from build123d import *

# Parameters (mm, degrees)
SKETCH1_W                                        = 32
SKETCH1_H                                        = 60
BOSS_EXTRUDE1_DEPTH                              = 7
SKETCH2_W                                        = 51
SKETCH2_H                                        = 8.75
CUT_EXTRUDE1_DEPTH                               = 65.078077374
CUT_EXTRUDE2_DEPTH                               = 65.078077374
F_10_0_10_DIAMETER_HOLE1_D                       = 10
F_10_0_10_DIAMETER_HOLE1_DEPTH                   = 14
M4X0_7_TAPPED_HOLE1_D                            = 2.1
M4X0_7_TAPPED_HOLE1_DEPTH                        = 14
M4X0_7_TAPPED_HOLE1_CBORE_D                      = 4
M4X0_7_TAPPED_HOLE1_CBORE_DEPTH                  = 2
CBORE_FOR_M3_HEX_HEAD_MACHINE_SCREW1_D           = 3.2
CBORE_FOR_M3_HEX_HEAD_MACHINE_SCREW1_CBORE_D     = 10.2
CBORE_FOR_M3_HEX_HEAD_MACHINE_SCREW1_CBORE_DEPTH = 1
F_4_1_4_1_DIAMETER_HOLE1_D                       = 4.1
F_4_1_4_1_DIAMETER_HOLE1_DEPTH                   = 14
F_4_1_4_1_DIAMETER_HOLE2_D                       = 4.1
FILLET3_R                                        = 12
CUT_EXTRUDE3_DEPTH                               = 65.078077374
SKETCH24_W                                       = 59.877724024
SKETCH24_H                                       = 41.345566777
CUT_EXTRUDE4_DEPTH                               = 7


# Read off the part's stored shape, not the designer's step: Mirror1
with BuildPart() as part:
    # Sketch1 → Boss-Extrude1 (new body)
    with BuildSketch(Plane(origin=(-2, 0, 0), x_dir=(0, -1, 0), z_dir=(-1, 0, 0))):
        with Locations((-8, 29)):
            Rectangle(SKETCH1_W, SKETCH1_H)
    extrude(amount=-BOSS_EXTRUDE1_DEPTH)

    # Sketch2 → Cut-Extrude1 (cut, through all)
    with BuildSketch(Plane(origin=(5, 0, 0), x_dir=(0, 0, -1), z_dir=(1, 0, 0))):
        with Locations((-21.5, 19.625)):
            Rectangle(SKETCH2_W, SKETCH2_H)
    extrude(amount=-CUT_EXTRUDE1_DEPTH, mode=Mode.SUBTRACT)

    # Sketch3 → Cut-Extrude2 (cut, through all)
    with BuildSketch(Plane(origin=(5, 0, 0), x_dir=(0, 0, -1), z_dir=(1, 0, 0))):
        Polygon((4, 6.75), (-21, 6.75), (-23, 15.25), (4, 15.25), align=None)
    extrude(amount=-CUT_EXTRUDE2_DEPTH, mode=Mode.SUBTRACT)

    # Ø10.0 (10) Diameter Hole1
    with Locations(Plane.ZY.offset(2)):
        with Locations((28, 0)):
            Hole(F_10_0_10_DIAMETER_HOLE1_D / 2, depth=F_10_0_10_DIAMETER_HOLE1_DEPTH)

    # M4x0.7 Tapped Hole1
    with Locations(Plane.ZY.offset(2)):
        with Locations((38.968179165, 5), (51.718179165, -2.361215932), (51.718179165, 12.361215932)):
            CounterBoreHole(M4X0_7_TAPPED_HOLE1_D / 2, M4X0_7_TAPPED_HOLE1_CBORE_D / 2, M4X0_7_TAPPED_HOLE1_CBORE_DEPTH, depth=M4X0_7_TAPPED_HOLE1_DEPTH)

    # CBORE for M3 Hex Head Machine Screw1 (through all)
    with Locations(Plane(origin=(5, 0, 0), x_dir=(0, 0, -1), z_dir=(1, 0, 0))):
        with Locations((-47.468179165, 5)):
            CounterBoreHole(CBORE_FOR_M3_HEX_HEAD_MACHINE_SCREW1_D / 2, CBORE_FOR_M3_HEX_HEAD_MACHINE_SCREW1_CBORE_D / 2, CBORE_FOR_M3_HEX_HEAD_MACHINE_SCREW1_CBORE_DEPTH)

    # Ø4.1 (4.1) Diameter Hole1
    with Locations(Plane.ZY.offset(2)):
        with Locations((32, 12)):
            Hole(F_4_1_4_1_DIAMETER_HOLE1_D / 2, depth=F_4_1_4_1_DIAMETER_HOLE1_DEPTH)

    # Ø4.1 (4.1) Diameter Hole2 (through all)
    with Locations(Plane(origin=(5, 0, 0), x_dir=(0, 0, -1), z_dir=(1, 0, 0))):
        with Locations((-55, 20.5)):
            Hole(F_4_1_4_1_DIAMETER_HOLE2_D / 2)

    # Fillet3
    fillet3_edges = [part.edges().sort_by_distance(p)[0] for p in [
        (1.5, -8, 59),
    ]]
    fillet(fillet3_edges, radius=FILLET3_R)

    # Cut-Sweep1: sweep along a path in Sketch22
    with BuildLine(Plane.ZY.offset(2)) as cut_sweep1_path:
        Line((-1, -8), (-8.402067684, 9.870172191))
    # Sketch21 → Cut-Sweep1 (sweep, cut)
    with BuildSketch(Plane.XZ.offset(8)):
        Polygon((-2, 10), (0.25, 10), (-1, 7), (-2, 7), align=None)
        Polygon((4, 7), (5, 7), (5, 10), (2.75, 10), align=None)
    sweep(path=cut_sweep1_path.line, mode=Mode.SUBTRACT)

    # Sketch23 → Cut-Extrude3 (cut, through all)
    with BuildSketch(Plane.ZY.offset(2)):
        Polygon((-1, 6.75), (0.890349955, 6.75), (7, -8), (-1, -8), align=None)
    extrude(amount=-CUT_EXTRUDE3_DEPTH, mode=Mode.SUBTRACT)

    # Mirror1: part across plane


with BuildPart() as part_1:
    add(part.part)
    add(part.part.mirror(Plane.ZY.offset(-5)))

    # Sketch24 → Cut-Extrude4 (cut)
    with BuildSketch(Plane.ZY.offset(2)):
        with Locations((29.938862012, 9.46680503)):
            Rectangle(SKETCH24_W, SKETCH24_H)
    extrude(amount=-CUT_EXTRUDE4_DEPTH, mode=Mode.SUBTRACT)


solid = part_1.part
Part model, mm, in its own coordinate system. A direction names the side the tool comes from. Give positions to 0.01 mm unless a question says otherwise; leave off trailing zeros. Write each loop counter-clockwise with the first axis right and the second up, starting at its lowest first coordinate (ties: lowest second). Pieces come first, ordered by that corner, then holes.
1) Cut at C-C on y = 9. Write the cut outline in (x, z), then the cut area to 3 significant figures.
Resolved:
outline: (5, 21.53) - (12, 21.53) - (12, 59) - (5, 59) - (5, 50.63) - (6, 50.63) - (6, 44.3) - (5, 44.3) - close
area: 256 mm2
2) Which spindle directions (+Z, -Z, +X, -X, +Y, -Y) get a long thin tool onto all of the face, cutting with end or side? Do faces 1 (the face through (10.384, -0.522, 5.381)), 2 (the face through (8.55, 20.59, 52.95)), 3 (the face through (5.493, 8.447, 51.227)). Say none if no direction does.
Resolved:
face 1: +X
face 2: +X, -X
face 3: -X
3) Cut at B-B on z = 55. Write the cut outline in (x, y), then the cut area to 3 significant figures.
Resolved:
outline: (5, -4.94) - (12, -4.94) - (12, 18.45) - (5, 18.45) - close; (5, 22.55) - (12, 22.55) - (12, 24) - (5, 24) - close
area: 174 mm2
4) Cut at A-A on z = 32. Write the cut outline in (x, y).
Resolved:
outline: (5, -8) - (12, -8) - (12, -3) - (5, -3) - close; (5, 3) - (12, 3) - (12, 9.95) - (5, 9.95) - close; (5, 14.05) - (12, 14.05) - (12, 15.25) - (5, 15.25) - close
5) Pin check, flat tips, straight feed: pin 1 (5 mm diameter, centred on y = 6.5, z = 45.5, fed in from -X); pin 2 (2.5 mm diameter, centred on y = -2.36, z = 51.72, fed in from +X); pin 3 (2 mm diameter, centred on x = 6.5, z = 41.5, fed in from +Y). Stop position of each tip, or through.
Resolved:
pin 1: stops at x = 6
pin 2: stops at x = 10
pin 3: stops at y = 15.25
6) Probe L1, parallel to Z at x = 11.5, y = 13; L2, parallel to Y at x = 5.75, z = 39; L3, parallel to Y at x = 9.25, z = 56.5. List the from-to ranges inside material, lowest first.
Resolved:
L1: z = 22.47 to 30.21, 33.79 to 49.82, 53.61 to 59
L2: y = -8 to 3.95, 6.05 to 15.25
L3: y = -3.33 to 19.1, 21.9 to 24
7) Two-plate mould, pull along Z, no slides. Class faces 4 (the face through (7.465, -2.046, 50.717)), 5 (the face through (8, 20, 47)), 6 (the face through (8.45, -4.39, 55.58)): released by +Z, released by -Z, zero draft, split by the parting line, or undercut.
Resolved:
face 4: undercut
face 5: released by -Z
face 6: released by +Z
8) Cut at D-D on z = 12.5. Write the cut outline in (x, y).
Resolved:
outline: (5, -8) - (12, -8) - (12, 6.75) - (5, 6.75) - close
